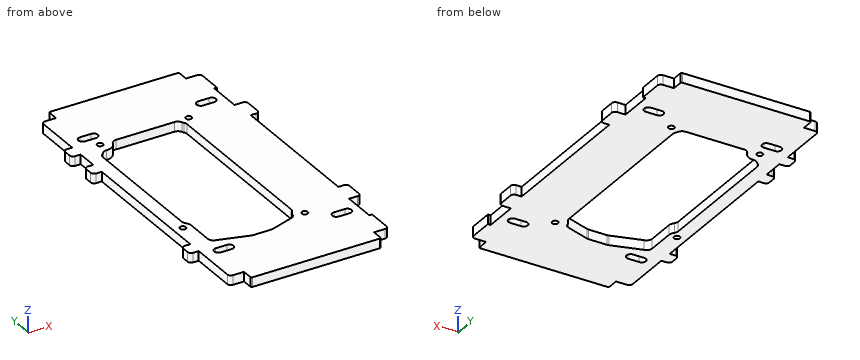
from build123d import *

# Parameters (mm, degrees)
SKETCH1_R           = 2.125
BOSS_EXTRUDE1_DEPTH = 6.88


with BuildPart() as part:
    # Sketch1 → Boss-Extrude1 (new body)
    with BuildSketch(Plane.XY):
        with BuildLine():
            Line((-78.364802088, -42.778869258), (-82.364802088, -42.778869258))
            ThreePointArc((-82.364802088, -42.778869258), (-84.132569041, -42.046636211), (-84.864802088, -40.278869258))
            Line((-84.864802088, -40.278869258), (-84.864802088, -35.278869258))
            ThreePointArc((-84.864802088, -35.278869258), (-84.132569041, -33.511102306), (-82.364802088, -32.778869258))
            Line((-82.364802088, -32.778869258), (-78.364802088, -32.778869258))
            Line((-78.364802088, -32.778869258), (-78.364802088, 72.221130742))
            Line((-78.364802088, 72.221130742), (-82.364802088, 72.221130742))
            ThreePointArc((-82.364802088, 72.221130742), (-84.132569041, 72.953363789), (-84.864802088, 74.721130742))
            Line((-84.864802088, 74.721130742), (-84.864802088, 79.721130742))
            ThreePointArc((-84.864802088, 79.721130742), (-84.132569041, 81.488897694), (-82.364802088, 82.221130742))
            Line((-82.364802088, 82.221130742), (-78.364802088, 82.221130742))
            Line((-78.364802088, 82.221130742), (-78.364802088, 97.221130742))
            Line((-78.364802088, 97.221130742), (-82.364802088, 97.221130742))
            ThreePointArc((-82.364802088, 97.221130742), (-84.132569041, 97.953363789), (-84.864802088, 99.721130742))
            Line((-84.864802088, 99.721130742), (-84.864802088, 104.721130742))
            ThreePointArc((-84.864802088, 104.721130742), (-84.132569041, 106.488897694), (-82.364802088, 107.221130742))
            Line((-82.364802088, 107.221130742), (-78.364802088, 107.221130742))
            Line((-78.364802088, 107.221130742), (-78.364802088, 141.221127314))
            ThreePointArc((-78.364802088, 141.221127314), (-77.632570253, 142.988896483), (-75.864802088, 143.721130742))
            Line((-75.864802088, 143.721130742), (-67.864802088, 143.721130742))
            Line((-67.864802088, 143.721130742), (-67.864802088, 151.221130742))
            ThreePointArc((-67.864802088, 151.221130742), (-67.571908869, 151.928237523), (-66.864802088, 152.221130742))
            Line((-66.864802088, 152.221130742), (25.135197912, 152.221130742))
            ThreePointArc((25.135197912, 152.221130742), (25.842304693, 151.928237523), (26.135197912, 151.221130742))
            Line((26.135197912, 151.221130742), (26.135197912, 143.721130742))
            Line((26.135197912, 143.721130742), (34.135197912, 143.721130742))
            ThreePointArc((34.135197912, 143.721130742), (35.902964865, 142.988897694), (36.635197912, 141.221130742))
            Line((36.635197912, 141.221130742), (36.635197912, 124.221130742))
            Line((36.635197912, 124.221130742), (34.635197912, 124.221130742))
            Line((34.635197912, 124.221130742), (34.635197912, 100.221130742))
            Line((34.635197912, 100.221130742), (40.635197912, 100.221130742))
            ThreePointArc((40.635197912, 100.221130742), (42.402964865, 99.488897694), (43.135197912, 97.721130742))
            Line((43.135197912, 97.721130742), (43.135197912, 86.721130742))
            ThreePointArc((43.135197912, 86.721130742), (42.402964865, 84.953363789), (40.635197912, 84.221130742))
            Line((40.635197912, 84.221130742), (36.635197912, 84.221130742))
            Line((36.635197912, 84.221130742), (36.635197912, -19.778869258))
            Line((36.635197912, -19.778869258), (40.635197912, -19.778869258))
            ThreePointArc((40.635197912, -19.778869258), (42.402964865, -20.511102306), (43.135197912, -22.278869258))
            Line((43.135197912, -22.278869258), (43.135197912, -33.278869258))
            ThreePointArc((43.135197912, -33.278869258), (42.402964865, -35.046636211), (40.635197912, -35.778869258))
            Line((40.635197912, -35.778869258), (34.635197912, -35.778869258))
            Line((34.635197912, -35.778869258), (34.635197912, -59.778869258))
            Line((34.635197912, -59.778869258), (36.635197912, -59.778869258))
            Line((36.635197912, -59.778869258), (36.635197912, -76.778869258))
            ThreePointArc((36.635197912, -76.778869258), (35.902964865, -78.546636211), (34.135197912, -79.278869258))
            Line((34.135197912, -79.278869258), (26.135197912, -79.278869258))
            Line((26.135197912, -79.278869258), (26.135197912, -86.778869258))
            ThreePointArc((26.135197912, -86.778869258), (25.842304693, -87.48597604), (25.135197912, -87.778869258))
            Line((25.135197912, -87.778869258), (-66.864802088, -87.778869258))
            ThreePointArc((-66.864802088, -87.778869258), (-67.571908869, -87.48597604), (-67.864802088, -86.778869258))
            Line((-67.864802088, -86.778869258), (-67.864802088, -79.278869258))
            Line((-67.864802088, -79.278869258), (-75.864802088, -79.278869258))
            ThreePointArc((-75.864802088, -79.278869258), (-77.632569041, -78.546636211), (-78.364802088, -76.778869258))
            Line((-78.364802088, -76.778869258), (-78.364802088, -42.778869258))
        make_face()
        with Locations((-71.704802088, -13.178869258)):
            Circle(SKETCH1_R, mode=Mode.SUBTRACT)
        with Locations((2.277397912, 101.421130742)):
            Circle(SKETCH1_R, mode=Mode.SUBTRACT)
        with Locations((-61.722602088, 101.421130741)):
            Circle(SKETCH1_R, mode=Mode.SUBTRACT)
        with Locations((2.277397912, -36.378869258)):
            Circle(SKETCH1_R, mode=Mode.SUBTRACT)
        with BuildLine():
            Line((17.827855969, -45.278869258), (25.827855969, -45.278869258))
            ThreePointArc((25.827855969, -45.278869258), (28.827855969, -48.278869258), (25.827855969, -51.278869258))
            Line((25.827855969, -51.278869258), (17.827855969, -51.278869258))
            ThreePointArc((17.827855969, -51.278869258), (14.827855969, -48.278869258), (17.827855969, -45.278869258))
        make_face(mode=Mode.SUBTRACT)
        with BuildLine():
            Line((-65.704802088, -13.178869258), (-65.704802088, -32.824689972))
            ThreePointArc((-65.704802088, -32.824689972), (-64.73917528, -35.430947697), (-62.308512422, -36.778869258))
            Line((-62.308512422, -36.778869258), (-40.709388186, -43.22032523))
            ThreePointArc((-40.709388186, -43.22032523), (-40.143864213, -43.345228063), (-39.566230949, -43.387155324))
            Line((-39.566230949, -43.387155324), (-26.151305592, -43.387155324))
            ThreePointArc((-26.151305592, -43.387155324), (-25.50948768, -43.33532829), (-24.884301528, -43.181190208))
            Line((-24.884301528, -43.181190208), (-8.176926635, -37.601823511))
            ThreePointArc((-8.176926635, -37.601823511), (-6.469142152, -36.4818554), (-5.536821161, -34.664815504))
            ThreePointArc((-5.536821161, -34.664815504), (-4.857565105, -32.760540535), (-3.722602088, -31.087366636))
            ThreePointArc((-3.722602088, -31.087366636), (-2.980944701, -29.855828888), (-2.722602088, -28.441615325))
            Line((-2.722602088, -28.441615325), (-2.722602088, 95.096575421))
            ThreePointArc((-2.722602088, 95.096575421), (-2.908751731, 96.3026208), (-3.449874815, 97.396413719))
            ThreePointArc((-3.449874815, 97.396413719), (-3.891134752, 98.112172481), (-4.243388939, 98.875676196))
            ThreePointArc((-4.243388939, 98.875676196), (-5.713248555, 100.724022037), (-7.969552854, 101.421130741))
            Line((-7.969552854, 101.421130741), (-50.408893589, 101.421130741))
            ThreePointArc((-50.408893589, 101.421130741), (-52.718294666, 100.687117065), (-54.180129755, 98.754464075))
            ThreePointArc((-54.180129755, 98.754464075), (-57.229450027, 94.802098746), (-62.028259496, 93.426972027))
            ThreePointArc((-62.028259496, 93.426972027), (-63.640931937, 93.153984004), (-65.009515325, 92.258319795))
            Line((-65.009515325, 92.258319795), (-67.193229213, 90.074605907))
            ThreePointArc((-67.193229213, 90.074605907), (-68.060320218, 88.776912512), (-68.364802088, 87.246178782))
            Line((-68.364802088, 87.246178782), (-68.364802088, -6.387374578))
            ThreePointArc((-68.364802088, -6.387374578), (-68.089315479, -7.84614118), (-67.300802088, -9.10397245))
            ThreePointArc((-67.300802088, -9.10397245), (-66.118032001, -10.990719355), (-65.704802088, -13.178869258))
        make_face(mode=Mode.SUBTRACT)
        with BuildLine():
            Line((-67.557460145, 109.721130742), (-59.557460145, 109.721130742))
            ThreePointArc((-59.557460145, 109.721130742), (-56.557460145, 112.721130742), (-59.557460145, 115.721130742))
            Line((-59.557460145, 115.721130742), (-67.557460145, 115.721130742))
            ThreePointArc((-67.557460145, 115.721130742), (-70.557460145, 112.721130742), (-67.557460145, 109.721130742))
        make_face(mode=Mode.SUBTRACT)
        with BuildLine():
            Line((17.827855969, 109.721130742), (25.827855969, 109.721130742))
            ThreePointArc((25.827855969, 109.721130742), (28.827855969, 112.721130742), (25.827855969, 115.721130742))
            Line((25.827855969, 115.721130742), (17.827855969, 115.721130742))
            ThreePointArc((17.827855969, 115.721130742), (14.827855969, 112.721130742), (17.827855969, 109.721130742))
        make_face(mode=Mode.SUBTRACT)
        with BuildLine():
            Line((-67.557460145, -45.278869258), (-59.557460145, -45.278869258))
            ThreePointArc((-59.557460145, -45.278869258), (-56.557460145, -48.278869258), (-59.557460145, -51.278869258))
            Line((-59.557460145, -51.278869258), (-67.557460145, -51.278869258))
            ThreePointArc((-67.557460145, -51.278869258), (-70.557460145, -48.278869258), (-67.557460145, -45.278869258))
        make_face(mode=Mode.SUBTRACT)
    extrude(amount=BOSS_EXTRUDE1_DEPTH)


solid = part.part
Design review of the part built by this model. Coordinates are the model's own, in mm. Give positions to 0.01 mm unless a question says otherwise; leave off trailing zeros. Loops run counter-clockwise (first coordinate to the right, second up) from the corner with the lowest first, then second, coordinate; pieces in that order, holes last. Notation, with made-up numbers: (53.5, 24.25) -> (73.5, 24.25) arc R15 cw to (73.5, 47.25) -> close; hole circle Ø10 at (7.5, 34.25). An arc over 180 degrees is marked (long way). One line per question, with ' | ' between items. Start each with the question number.
(1) We need section C-C (z = 5.5). State how many separate pieces and enclosed holes the cut face has, and give its area (3 significant figures).
(2) We need section A-A (y = 23). State the section outline as (x, z) points, and give its area (3 significant figures).
(3) We need section B-B (x = -16.5). State the section outline as (y, z) points.
(4) We need section D-D (y = 129). State the section outline as (x, z) points, and give its area (3 significant figures).
(5) Insertion check: P1, Ø1, axis at y = 5, z = 1.5, coming from the +X side; P2, Ø3.5, axis at x = 32, z = 4.5, coming from the -Y side; P3, Ø2, axis at x = -80, z = 3, coming from the -Y side. Each pin has a flat end and moves straight along its axis. Give the tip position at first contact, or say it passes through.
(6) For line 1 (Y direction, x = 21.5, z = 2.75); line 2 (X direction, y = 15, z = 5); line 3 (Y direction, x = -61, z = 3.75), list the stretches that pass through material, from the lowest coordinate up.
The answers:
1) separate pieces: 1 | enclosed holes: 9 | area: 18,100 mm^2
2) outline: (-78.36, 0) -> (-68.36, 0) -> (-68.36, 6.88) -> (-78.36, 6.88) -> close; (-2.72, 0) -> (36.64, 0) -> (36.64, 6.88) -> (-2.72, 6.88) -> close | area: 340 mm^2
3) outline: (-87.78, 0) -> (-40.38, 0) -> (-40.38, 6.88) -> (-87.78, 6.88) -> close; (101.42, 0) -> (152.22, 0) -> (152.22, 6.88) -> (101.42, 6.88) -> close
4) outline: (-78.36, 0) -> (36.64, 0) -> (36.64, 6.88) -> (-78.36, 6.88) -> close | area: 791 mm^2
5) P1: stops at x = 36.64 | P2: stops at y = -79.28 | P3: stops at y = -42.78
6) line 1: y = -87.78 to -51.28, -45.28 to 109.72, 115.72 to 152.22 | line 2: x = -78.36 to -68.36, -2.72 to 36.64 | line 3: y = -87.78 to -51.28, -45.28 to -37.17, 93.45 to 99.42, 103.42 to 109.72, 115.72 to 152.22
